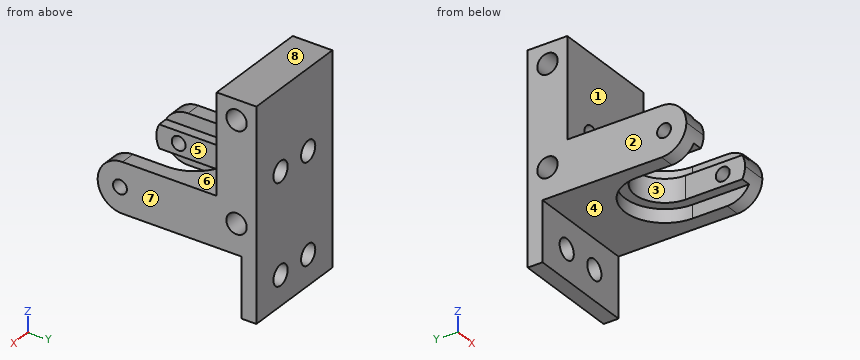
```python
from build123d import *

# Parameters (mm, degrees)
F0_W     = 22
F0_H     = 42
F1_DEPTH = 3
F2_W     = 3
F2_H     = 30
F2_W_2   = 5
F3_DEPTH = 22
F4_D     = 4.1
F7_DEPTH = 5
F8_DEPTH = 2.325
F9_R     = 4.99999
F11_D    = 4.1
F12_D    = 2.8


# Not quite as in the source:
# - a fillet or chamfer is up to 0.001 mm smaller than in the source, because OpenCascade refuses the exact size


with BuildPart() as f1:
    # F0 (on Front) → F1 (new body)
    with BuildSketch(Plane.XZ):
        with Locations((-28.9233987555, 27.9422005266)):
            Rectangle(F0_W, F0_H)
    extrude(amount=F1_DEPTH)

    # F2 (on face) → F3 (join)
    with BuildSketch(Plane(origin=(-39.9233987555, 0, 0), x_dir=(0, -1, 0), z_dir=(-1, 0, 0))):
        with Locations((1.5, 33.9422005266)):
            Rectangle(F2_W, F2_H)
        with Locations((5.5, 33.9422005266)):
            Rectangle(F2_W_2, F2_H)
    extrude(amount=-F3_DEPTH)

    # F4 (through all)
    with Locations(Plane(origin=(0, 0, 0), x_dir=(1, 0, 0), z_dir=(0, 1, 0))):
        with Locations((-24.9233987555, -12.9422005266), (-32.9233987555, -12.9422005266), (-32.9233987555, -32.9422005266), (-24.9233987555, -32.9422005266)):
            Hole(F4_D / 2)

    # F6 (on line) → F7 (join, symmetric)
    with BuildSketch(Plane.XY.offset(23.9422005266)):
        with BuildLine():
            ThreePointArc((-36.9233987555, -20), (-28.9233987555, -12), (-20.9233987555, -20))
            Line((-20.9233987555, -20), (-20.9233987555, -32))
            Line((-20.9233987555, -32), (-17.9233987555, -32))
            Line((-17.9233987555, -32), (-17.9233987555, 0))
            Line((-17.9233987555, 0), (-39.9233987555, 0))
            Line((-39.9233987555, 0), (-39.9233987555, -32))
            Line((-39.9233987555, -32), (-36.9233987555, -32))
            Line((-36.9233987555, -32), (-36.9233987555, -20))
        make_face()
    extrude(amount=F7_DEPTH, both=True)

    # F6 (on line) → F8 (join, symmetric)
    with BuildSketch(Plane.XY.offset(23.9422005266)):
        with BuildLine():
            ThreePointArc((-34.9233987555, -20), (-28.9233987555, -14), (-22.9233987555, -20))
            Line((-22.9233987555, -20), (-22.9233987555, -25.2915026221))
            ThreePointArc((-22.9233987555, -25.2915026221), (-21.4400839819, -22.8284271247), (-20.9233987555, -20))
            ThreePointArc((-20.9233987555, -20), (-28.9233987555, -12), (-36.9233987555, -20))
            ThreePointArc((-36.9233987555, -20), (-36.406713529, -22.8284271247), (-34.9233987555, -25.2915026221))
            Line((-34.9233987555, -25.2915026221), (-34.9233987555, -20))
        make_face()
        with BuildLine():
            Line((-34.9233987555, -32), (-34.9233987555, -25.2915026221))
            ThreePointArc((-34.9233987555, -25.2915026221), (-36.406713529, -22.8284271247), (-36.9233987555, -20))
            Line((-36.9233987555, -20), (-36.9233987555, -32))
            Line((-36.9233987555, -32), (-34.9233987555, -32))
        make_face()
        with BuildLine():
            ThreePointArc((-20.9233987555, -20), (-21.4400839819, -22.8284271247), (-22.9233987555, -25.2915026221))
            Line((-22.9233987555, -25.2915026221), (-22.9233987555, -32))
            Line((-22.9233987555, -32), (-20.9233987555, -32))
            Line((-20.9233987555, -32), (-20.9233987555, -20))
        make_face()
    extrude(amount=F8_DEPTH, both=True)

    # F9 (radius 5 in the source; OpenCascade refuses exactly that, so slightly less here)
    f9_edges = [f1.edges().sort_by_distance(p)[0] for p in [
        (-38.423399, -32, 28.942201),
        (-38.423399, -32, 18.942201),
        (-19.423399, -32, 18.942201),
        (-19.423399, -32, 28.942201),
    ]]
    fillet(f9_edges, radius=F9_R)

    # F11 (through all)
    with Locations(Plane(origin=(-39.9233987555, 0, 0), x_dir=(0, -1, 0), z_dir=(-1, 0, 0))):
        with Locations((4, 44.9422005266), (4, 24.9422005266)):
            Hole(F11_D / 2)

    # F12 (through all)
    with Locations(Plane(origin=(-39.9233987555, 0, 0), x_dir=(0, -1, 0), z_dir=(-1, 0, 0))):
        with Locations((27.5, 23.9422005266)):
            Hole(F12_D / 2)


solid = f1.part
```
Check sheet for the modelled part. Datum: model origin and axes. Units: mm. Face numbers are marked on the shaded views. A direction names the side the tool comes from. Coordinates: 2 decimals unless noted, no trailing zeros. Loops run counter-clockwise (first coordinate to the right, second up) from the corner with the lowest first, then second, coordinate; pieces in that order, holes last.
1) Sectioned sample at C-C (z = 32). Record the boundary of the cut face in (x, y), and give its area (3 significant figures).
2) Sectioned sample at A-A (x = -26.25). Record the boundary of the cut face in (y, z).
3) Sectioned sample at B-B (y = -4). Record the boundary of the cut face in (x, z), and give its area (3 significant figures).
4) Material ranges on probe 1 along Z at (x, y) = (-30.25, -4); probe 2 along Y at (x, z) = (-35, 30); probe 3 along Y at (x, z) = (-26.5, 25), recorded low to high.
5) Access from +Z, -Z, +X, -X, +Y, -Y to the whole of each face (thin tool, end or side, straight path). Record for the marked faces 4, 5, 6, 7 and 8.
6) Release check for a two-part mould opening along X. For the marked faces 1, 2 and 3 record: released by +X, released by -X, zero draft, split by the parting line, or undercut.
7) Sectioned sample at D-D (y = -27.5). Record the boundary of the cut face in (x, z), and give its area (3 significant figures).
8) Gauge pin test, flat ends, axial feed: pin 1 (3.5 mm diameter, centred on y = -4, z = 44.94, fed in from -X); pin 2 (10 mm diameter, centred on x = -31.5, y = -20, fed in from +Z); pin 3 (12 mm diameter, centred on x = -23, z = 40, fed in from -Y); pin 4 (1 mm diameter, centred on x = -34.5, y = -12, fed in from -Z). Record the tip position at first contact, or that the pin passes through.
Check sheet entries:
1. outline: (-39.92, -8) - (-34.74, -8) - (-34.74, 0) - (-39.92, 0) - close; (-31.1, -8) - (-26.74, -8) - (-26.74, 0) - (-31.1, 0) - close; (-23.1, -8) - (-17.92, -8) - (-17.92, 0) - (-23.1, 0) - close
1. area: 118 mm2
2. outline: (-14.63, 21.62) - (-12.46, 21.62) - (-12.46, 18.94) - (-3, 18.94) - (-3, 14.51) - (0, 14.51) - (0, 31.38) - (-8, 31.38) - (-8, 28.94) - (-12.46, 28.94) - (-12.46, 26.27) - (-14.63, 26.27) - close; (-8, 34.51) - (0, 34.51) - (0, 48.94) - (-8, 48.94) - close; (-3, 6.94) - (0, 6.94) - (0, 11.38) - (-3, 11.38) - close; hole circle Ø4.1 at (-4, 24.94); hole circle Ø4.1 at (-4, 44.94)
3. outline: (-39.92, 18.94) - (-17.92, 18.94) - (-17.92, 22.89) - (-39.92, 22.89) - close; (-39.92, 26.99) - (-17.92, 26.99) - (-17.92, 42.89) - (-39.92, 42.89) - close; (-39.92, 46.99) - (-17.92, 46.99) - (-17.92, 48.94) - (-39.92, 48.94) - close; hole circle Ø4.1 at (-32.92, 32.94); hole circle Ø4.1 at (-24.92, 32.94)
3. area: 453 mm2
4. probe 1: z = 18.94 to 22.89, 26.99 to 42.89, 46.99 to 48.94
4. probe 2: y = -8 to 0
4. probe 3: y = -14.51 to -6.05, -1.95 to 0
5. face 4: -Z, +X, -X, -Y
5. face 5: +Z, -Z, -Y
5. face 6: +Z, +X, -X, -Y
5. face 7: +Z, -Z, +X, +Y, -Y
5. face 8: +Z, +X, -X, +Y, -Y
6. face 1: zero draft
6. face 2: released by -X
6. face 3: undercut
7. outline: (-39.92, 18.97) - (-36.92, 18.97) - (-36.92, 21.62) - (-34.92, 21.62) - (-34.92, 22.54) - (-39.92, 22.54) - close; (-39.92, 25.34) - (-34.92, 25.34) - (-34.92, 26.27) - (-36.92, 26.27) - (-36.92, 28.92) - (-39.92, 28.92) - close; (-22.92, 21.62) - (-20.92, 21.62) - (-20.92, 18.97) - (-17.92, 18.97) - (-17.92, 22.54) - (-22.92, 22.54) - close; (-22.92, 25.34) - (-17.92, 25.34) - (-17.92, 28.92) - (-20.92, 28.92) - (-20.92, 26.27) - (-22.92, 26.27) - close
7. area: 50.3 mm2
8. pin 1: passes through
8. pin 2: stops at z = 26.27
8. pin 3: stops at y = -8
8. pin 4: stops at z = 18.94
